Autodesk Inventor part; units mm, degrees
ref_plane "YZ Plane" through (0, 0, 0) normal (1, 0, 0) x (0, 1, 0)
ref_plane "XZ Plane" through (0, 0, 0) normal (0, 1, 0) x (-1, 0, 0)
ref_plane "XY Plane" through (0, 0, 0) normal (0, 0, 1) x (1, 0, 0)
sketch "Sketch1" plane through (0, 0, 0) normal (0, 0, 1) x (1, 0, 0)
  circle A0 centre (-6.35, 152.4) radius 2.1844
  circle A1 centre (6.35, 152.4) radius 2.1844
  circle A2 centre (-6.35, 88.9) radius 2.1844
  circle A3 centre (6.35, 88.9) radius 2.1844
  arc A4 (-1.8034, 135.6614) -> (-2.3114, 135.1534) centre (-1.8034, 135.1534) ccw
  line L0 (-2.3114, 131.5466) -> (-2.3114, 135.1534)
  line L1 (-1.8034, 135.6614) -> (1.8034, 135.6614)
  arc A5 (-2.3114, 131.5466) -> (-1.8034, 131.0386) centre (-1.8034, 131.5466) ccw
  line L2 (1.8034, 131.0386) -> (-1.8034, 131.0386)
  arc A6 (1.8034, 131.0386) -> (2.3114, 131.5466) centre (1.8034, 131.5466) ccw
  line L3 (2.3114, 135.1534) -> (2.3114, 131.5466)
  arc A7 (2.3114, 135.1534) -> (1.8034, 135.6614) centre (1.8034, 135.1534) ccw
  circle A8 centre (0, 120.65) radius 2.1844
  circle A9 centre (0, 107.95) radius 6.35
  line L4 (36.7693, 131.7499) -> (36.7693, 177.9954)
  line L5 (-12.7, 88.9) -> (-12.7, 152.4)
  line L6 (-6.35, 82.55) -> (6.35, 82.55)
  spline S0 degree 4 poles (-12.7, 88.9) (-12.7, 87.6131) (-12.7, 85.0392) (-10.2108, 82.55) (-7.6369, 82.55) (-6.35, 82.55) knots 0 0 0 0 0 0.5 1 1 1 1 1
  spline S1 degree 4 poles (6.35, 82.55) (8.1081, 82.55) (9.8661, 82.55) (11.0889, 84.4373) (11.9675, 85.9392) knots 0 0 0 0 0 1 1 1 1 1
  line L7 (11.9675, 85.9392) -> (33.5511, 122.8344)
  spline S2 degree 4 poles (33.5511, 122.8344) (34.1544, 123.8656) (35.3609, 125.928) (36.7693, 128.0899) (36.7693, 130.5299) (36.7693, 131.7499) knots 0 0 0 0 0 0.5 1 1 1 1 1
  spline S3 degree 4 poles (-11.9358, 155.4201) (-12.0668, 155.0524) (-12.3287, 154.3171) (-12.7, 153.5861) (-12.7, 152.7954) (-12.7, 152.4) knots 0 0 0 0 0 0.5 1 1 1 1 1
  line L8 (-11.9358, 155.4201) -> (0, 188.9294)
  line L9 (18.2111, 198.8461) -> (35.8036, 182.8241)
  spline S4 degree 4 poles (0, 188.9294) (0.9805, 191.6822) (2.9416, 197.1879) (10.5283, 205.8431) (15.6502, 201.1784) (18.2111, 198.8461) knots 0 0 0 0 0 0.5 1 1 1 1 1
  spline S5 degree 4 poles (35.8036, 182.8241) (36.303, 182.3693) (37.3018, 181.4596) (36.7693, 179.86) (36.7693, 178.6169) (36.7693, 177.9954) knots 0 0 0 0 0 0.5 1 1 1 1 1
  circle A10 centre (21.7424, 190.5) radius 2.1844
  circle A11 centre (5.1816, 190.5) radius 2.1844
  point P0 (0, 0)
  point P1 (21.7424, 177.8)
  point P2 (14.224, 190.5)
  dimension "d1" = 4.3688
  dimension "d2" = 12.7
  dimension "d10" = 0
  dimension "d13" = 16.5608
  dimension "d16" = 12.7
  dimension "d17" = 7.5184
extrude "Extrusion1" add sketch "Sketch1" along normal blind 1.524
sketch "Sketch2" plane through (0, 0, 1.524) normal (0, 0, 1) x (1, 0, 0)
  line L0 (12.9318, 114.6329) -> (12.9318, 139.693) construction
  line L1 (12.9318, 139.693) -> (20.9407, 139.693) construction
  line L2 (20.9407, 139.693) -> (20.9407, 114.6329) construction
  line L3 (20.9407, 114.6329) -> (12.9318, 114.6329) construction
  line L4 (-6.35, 82.55) -> (6.35, 82.55)
  line L5 (11.9675, 85.9392) -> (33.5511, 122.8344)
  line L6 (36.7693, 131.7499) -> (36.7693, 177.9954)
  line L7 (35.8036, 182.8241) -> (18.2111, 198.8461)
  line L8 (0, 188.9294) -> (-11.9358, 155.4201)
  line L9 (-12.7, 152.4) -> (-12.7, 88.9)
  circle A0 centre (-6.35, 152.4) radius 2.1844
  circle A1 centre (6.35, 152.4) radius 2.1844
  circle A2 centre (6.35, 88.9) radius 2.1844
  circle A3 centre (0, 120.65) radius 2.1844
  circle A4 centre (0, 107.95) radius 6.35
  circle A5 centre (21.7424, 190.5) radius 2.1844
  circle A6 centre (5.1816, 190.5) radius 2.1844
  line L10 (2.3114, 135.1534) -> (2.3114, 131.5466)
  arc A7 (1.8034, 131.0386) -> (2.3114, 131.5466) centre (1.8034, 131.5466) ccw
  line L11 (1.8034, 131.0386) -> (-1.8034, 131.0386)
  arc A8 (-2.3114, 131.5466) -> (-1.8034, 131.0386) centre (-1.8034, 131.5466) ccw
  line L12 (-2.3114, 131.5466) -> (-2.3114, 135.1534)
  arc A9 (-1.8034, 135.6614) -> (-2.3114, 135.1534) centre (-1.8034, 135.1534) ccw
  line L13 (-1.8034, 135.6614) -> (1.8034, 135.6614)
  arc A10 (2.3114, 135.1534) -> (1.8034, 135.6614) centre (1.8034, 135.1534) ccw
  circle A11 centre (-6.35, 88.9) radius 2.1844
  point P0 (0, 0)
properties part number "sled"
Source: CAD feature listing. Evaluate the final solid. Frame: model axes, mm. Give positions to 0.01 mm unless a question says otherwise; leave off trailing zeros. Order: outer loops, then holes, each group sorted by start corner. A loop starts at its lowest first (then second) coordinate and runs counter-clockwise, first axis right, second up.
(1) Contact query for a flat-ended pin moving along its axis: P1, Ø0.5, axis at y = 156.5, z = 1, coming from the +X side. Output: stop coordinate, or through.
(2) Section query B-B (x = 21). Return the cut outline in (y, z), plus the area to 3 significant figures.
(3) Material intervals for line 1 along X through (y, z) = (152.4, 0.85); line 2 along X through (y, z) = (190.5, 1.2); line 3 along X through (y, z) = (122.5, 1.4), sorted ascending.
(4) Pull-direction query (Y, two-part tool) for faces 1 (the face through (-6.05, 171.94, 0.75)), 2 (the face through (12, 145, 1.524)), 3 (the face through (-1.38, 114.15, 0.75)); classes: +Y half, -Y half, draft (parallel to the pull), parting line (faces both ways), or undercut.
(5) Section query A-A (y = 113). Return the cut outline in (x, z), plus the area to 3 significant figures.
(6) Section query C-C (z = 0.8). State how many separate pieces and enclosed holes the cut face has, plus the area to 3 significant figures.
(7) Section query D-D (y = 99.5). Return the cut outline in (x, z), plus the area to 3 significant figures.
Outcome:
1. P1: stops at x = 36.77
2. outline: (101.38, 0) - (188.45, 0) - (188.45, 1.52) - (101.38, 1.52) - close; (192.55, 0) - (196.31, 0) - (196.31, 1.52) - (192.55, 1.52) - close
2. area: 138 mm2
3. line 1: x = -12.7 to -8.53, -4.17 to 4.17, 8.53 to 36.77
3. line 2: x = 0.57 to 3, 7.37 to 19.56, 23.93 to 27.38
3. line 3: x = -12.7 to -1.16, 1.16 to 33.36
4. face 1: +Y half
4. face 2: draft
4. face 3: undercut
5. outline: (-12.7, 0) - (-3.85, 0) - (-3.85, 1.52) - (-12.7, 1.52) - close; (3.85, 0) - (27.8, 0) - (27.8, 1.52) - (3.85, 1.52) - close
5. area: 50.0 mm2
6. separate pieces: 1
6. enclosed holes: 9
6. area: 4,370 mm2
7. outline: (-12.7, 0) - (19.9, 0) - (19.9, 1.52) - (-12.7, 1.52) - close
7. area: 49.7 mm2
